```python
from build123d import *

# Parameters (mm, degrees)
F2_R = 0.5
F3_R = 0.05


with BuildPart() as f1:
    # F0 (on Front) → F1 (revolve)
    with BuildSketch(Plane.XZ):
        Polygon((1.6, 3), (1.6, 0), (3, 0), (2.0743638743, 1.5), (3, 3), align=None)
    revolve(axis=Axis((0, 0, 1.4736446901), (0, 0, -1)))

    # F2
    f2_edges = [f1.edges().sort_by_distance(p)[0] for p in [
        (-1.6, 0, 3),
        (-1.6, 0, 0),
    ]]
    fillet(f2_edges, radius=F2_R)

    # F3
    f3_edges = [f1.edges().sort_by_distance(p)[0] for p in [
        (-3, 0, 3),
        (-3, 0, 0),
    ]]
    fillet(f3_edges, radius=F3_R)


solid = f1.part
```
Check sheet for the modelled part. Datum: model origin and axes. Units: mm. Round coordinates to 2 decimals unless told otherwise and drop trailing zeros. Loops run counter-clockwise (first coordinate to the right, second up) from the corner with the lowest first, then second, coordinate; pieces in that order, holes last. Notation, with made-up numbers: (-4, 42.25) -> (47, 42.25) arc R35 ccw to (47, 76.25) -> close; hole circle Ø1 at (60, 53). An arc over 180 degrees is marked (long way). Answer in a Markdown table with one row per item.
Q1. Thickness scan on L1, parallel to X at y = 0, z = 2; L2, parallel to Y at x = 0, z = 1.35; L3, parallel to X at y = 0, z = 1.9. Record the ranges inside material, lowest first.
Data:
| item | result |
|---|---|
| L1 | x = -2.38 to -1.6, 1.6 to 2.38 |
| L2 | y = -2.17 to -1.6, 1.6 to 2.17 |
| L3 | x = -2.32 to -1.6, 1.6 to 2.32 |
Q2. Sectioned sample at D-D on z = 0.95. Enter the section's corners in (x, y).
Data:
| item | result |
|---|---|
| outline | circle Ø4.83 at (0, 0); hole circle Ø3.2 at (0, 0) |
Q3. Sectioned sample at C-C on z = 1.35. Enter the section's corners in (x, y), then the cut area to 3 significant figures.
Data:
| item | result |
|---|---|
| outline | circle Ø4.33 at (0, 0); hole circle Ø3.2 at (0, 0) |
| area | 6.71 mm^2 |
Q4. Sectioned sample at A-A on x = 0. Enter the section's corners in (y, z), then the cut area to 3 significant figures.
Data:
| item | result |
|---|---|
| outline | (-2.95, 0.08) arc R0.05 ccw to (-2.91, 0) -> (-2.1, 0) arc R0.5 ccw to (-1.6, 0.5) -> (-1.6, 2.5) arc R0.5 ccw to (-2.1, 3) -> (-2.91, 3) arc R0.05 ccw to (-2.95, 2.92) -> (-2.07, 1.5) -> close; (1.6, 0.5) arc R0.5 ccw to (2.1, 0) -> (2.91, 0) arc R0.05 ccw to (2.95, 0.08) -> (2.07, 1.5) -> (2.95, 2.92) arc R0.05 ccw to (2.91, 3) -> (2.1, 3) arc R0.5 ccw to (1.6, 2.5) -> close |
| area | 5.40 mm^2 |
Q5. Go/stop test with flat-tipped pins: P1, Ø1, axis at x = 1, z = 1.5, coming from the +Y side; P2, Ø3, axis at x = 0, y = 0, coming from the -Z side; P3, Ø1, axis at x = -1, z = 2.5, coming from the -Y side. Record where each tip stops, or that it passes through.
Data:
| item | result |
|---|---|
| P1 | stops at y = 2.22 |
| P2 | passes through |
| P3 | stops at y = -2.86 |
